from build123d import *

# Parameters (mm, degrees)
SKETCH1_R                    = 75.819
SKETCH1_R_2                  = 48.387
BOSS_EXTRUDE1_DEPTH          = 19.812
SKETCH2_R                    = 50.927
CUT_EXTRUDE1_DEPTH           = 8.7122
CHAMFER1_SIZE                = 0.762
SKETCH4_R                    = 4.2164
CUT_EXTRUDE2_DEPTH           = 20.812
CHAMFER2_SIZE                = 0.381
CIRPATTERN1_COUNT            = 16
CHAMFER2_OF_CIRPATTERN1_SIZE = 0.381
CUT_EXTRUDE3_DEPTH           = 0.79375


with BuildPart() as part:
    # Sketch1 → Boss-Extrude1 (new body)
    with BuildSketch(Plane(origin=(0, 0, 0), x_dir=(1, 0, 0), z_dir=(0, 1, 0))):
        Circle(SKETCH1_R)
        Circle(SKETCH1_R_2, mode=Mode.SUBTRACT)
    extrude(amount=BOSS_EXTRUDE1_DEPTH)

    # Sketch2 → Cut-Extrude1 (cut)
    with BuildSketch(Plane(origin=(0, 19.812, 0), x_dir=(1, 0, 0), z_dir=(0, 1, 0))):
        Circle(SKETCH2_R)
    extrude(amount=-CUT_EXTRUDE1_DEPTH, mode=Mode.SUBTRACT)

    # Chamfer1
    chamfer1_edges = [part.edges().sort_by_distance(p)[0] for p in [
        (-50.927, 19.812, 0),
        (-75.819, 0, 0),
        (-75.819, 19.812, 0),
    ]]
    chamfer(chamfer1_edges, length=CHAMFER1_SIZE)

    # Sketch3 → Cut-Revolve1 (revolve, cut)
    with BuildSketch(Plane.XY):
        Polygon((-60.325, 0), (-60.325, 1.6256), (-57.658, 0.6604), (-57.658, 1.27), (0, 1.27), (0, 0), align=None)
    revolve(axis=Axis((0, 19.812, 0), (0, -1, 0)), mode=Mode.SUBTRACT)

    # Sketch4 → Cut-Extrude2 (cut, through all)
    with BuildSketch(Plane(origin=(0, 19.812, 0), x_dir=(1, 0, 0), z_dir=(0, 1, 0))):
        with Locations((-12.705374275, 63.874229857)):
            Circle(SKETCH4_R)
    cut_extrude2 = extrude(amount=-CUT_EXTRUDE2_DEPTH, mode=Mode.SUBTRACT)

    # Chamfer2
    chamfer2_edges = [part.edges().sort_by_distance(p)[0] for p in [
        (-16.921774275, 0, -63.874229857),
        (-16.921774275, 19.812, -63.874229857),
    ]]
    chamfer(chamfer2_edges, length=CHAMFER2_SIZE)

    # CirPattern1: Cut-Extrude2 ×16 about axis
    cirpattern1_axis = Axis((0, 0, 0), (0, 1, 0))
    for i in range(1, CIRPATTERN1_COUNT):
        add(cut_extrude2.rotate(cirpattern1_axis, i * 360 / CIRPATTERN1_COUNT), mode=Mode.SUBTRACT)

    # Chamfer2 of CirPattern1
    chamfer2_of_cirpattern1_edges = [part.edges().sort_by_distance(p)[0] for p in [
        (-40.077290428, 0, -52.536410959),
        (-40.077290428, 19.812, -52.536410959),
        (-57.131402415, 0, -33.200399735),
        (-57.131402415, 19.812, -33.200399735),
        (-65.487776282, 0, -8.809928615),
        (-65.487776282, 19.812, -8.809928615),
        (-63.874229857, 0, 16.921774275),
        (-63.874229857, 19.812, 16.921774275),
        (-52.536410959, 0, 40.077290428),
        (-52.536410959, 19.812, 40.077290428),
        (-33.200399735, 0, 57.131402415),
        (-33.200399735, 19.812, 57.131402415),
        (-8.809928615, 0, 65.487776282),
        (-8.809928615, 19.812, 65.487776282),
        (16.921774275, 0, 63.874229857),
        (16.921774275, 19.812, 63.874229857),
        (40.077290428, 0, 52.536410959),
        (40.077290428, 19.812, 52.536410959),
        (57.131402415, 0, 33.200399735),
        (57.131402415, 19.812, 33.200399735),
        (65.487776282, 0, 8.809928615),
        (65.487776282, 19.812, 8.809928615),
        (63.874229857, 0, -16.921774275),
        (63.874229857, 19.812, -16.921774275),
        (52.536410959, 0, -40.077290428),
        (52.536410959, 19.812, -40.077290428),
        (33.200399735, 0, -57.131402415),
        (33.200399735, 19.812, -57.131402415),
        (8.809928615, 0, -65.487776282),
        (8.809928615, 19.812, -65.487776282),
    ]]
    chamfer(chamfer2_of_cirpattern1_edges, length=CHAMFER2_OF_CIRPATTERN1_SIZE)

    # Sketch5 → Cut-Extrude3 (cut, symmetric)
    with BuildSketch(Plane.XY):
        Polygon((-59.310240326, 0.913241856), (-75.819, 1.778429289), (-75.819, -2.195076128), (-59.310240326, -2.195076128), align=None)
        Polygon((59.310240326, 0.913241856), (59.310240326, -2.195076128), (75.819, -2.195076128), (75.819, 1.778429289), align=None)
    extrude(amount=CUT_EXTRUDE3_DEPTH, both=True, mode=Mode.SUBTRACT)


solid = part.part
Here's how the part is built. I have some questions about the finished solid (model axes, mm). A direction names the side the tool comes from. Round coordinates to 2 decimals unless told otherwise and drop trailing zeros. Order: outer loops, then holes, each group sorted by start corner. A loop starts at its lowest first (then second) coordinate and runs counter-clockwise, first axis right, second up. Notation, with made-up numbers: (-1, 85) -> (9, 85) arc R13 ccw to (9, 107) -> close; hole circle Ø7 at (-7.75, -3.5). An arc over 180 degrees is marked (long way). Return JSON: item names as keys, results as strings.
Q1. If we section it at A-A on x = 0: List the corners of the cut face in (y, z) for me (3 decimals), plus the area to 3 significant figures.
Filled sheet:
{"outline": "(0, -75.057) -> (0.762, -75.819) -> (19.05, -75.819) -> (19.812, -75.057) -> (19.812, -51.689) -> (19.05, -50.927) -> (11.1, -50.927) -> (11.1, -48.387) -> (1.27, -48.387) -> (1.27, -57.658) -> (0.66, -57.658) -> (1.626, -60.325) -> (0, -60.325) -> close; (0, 60.325) -> (1.626, 60.325) -> (0.66, 57.658) -> (1.27, 57.658) -> (1.27, 48.387) -> (11.1, 48.387) -> (11.1, 50.927) -> (19.05, 50.927) -> (19.812, 51.689) -> (19.812, 75.057) -> (19.05, 75.819) -> (0.762, 75.819) -> (0, 75.057) -> close", "area": "1,010 mm^2"}
Q2. If we section it at B-B on y = 13.75: Give the number of separate pieces and of enclosed holes in the cut face, plus the area to 3 significant figures.
Filled sheet:
{"separate pieces": "1", "enclosed holes": "17", "area": "9,020 mm^2"}
Q3. Which directions (+Z, -Z, +X, -X, +Y, -Y) give clear straight access to the entire face, cutting with the end or side of a thin tool? Please do faces 1 (the cylindrical face through (12.499, 0.969, 56.287)), 2 (the cylindrical face through (34.91, 10.04, -50.13)).
Filled sheet:
{"face 1": "-Y", "face 2": "+Y, -Y"}
Q4. I need wall thicknesses on line 1 along Z through (x, y) = (9, 3.5); line 2 along Z through (x, y) = (-62.5, 9.75); line 3 along X through (y, z) = (13.5, 14.5). Which ranges of each line are inside material? Lowest first, please. Write a range as from..to.
Filled sheet:
{"line 1": "z = -75.28..-65.89, -61.86..-47.54, 47.54..61.86, 65.89..75.28", "line 2": "z = -42.92..-16.69, -8.72..8.72, 16.69..42.92", "line 3": "x = -74.42..-67.69, -60.06..-48.82, 48.82..60.06, 67.69..74.42"}
Q5. If we mould it in two halves opening along X, with no side actions, what happens to faces 3 (the cylindrical face through (-54.148, 10.039, 31.965)), 4 (the conical face through (-1.64, 0.12, 75.16)), 5 (the cylindrical face through (59.76, 10.04, -13.62)), 6 (the flat face through (0, 0, -63))? For each: released by +X, released by -X, zero draft, split by the parting line, or undercut.
Filled sheet:
{"face 3": "undercut", "face 4": "split by the parting line", "face 5": "undercut", "face 6": "zero draft"}
Q6. For pin 1 Ø2 at (y, z) = (15, 3) entering from +X; pin 2 Ø13.5 at (x, z) = (-12.71, -63.87) entering from -Y; pin 3 Ø1.5 at (y, z) = (14, -27) entering from -X; pin 4 Ø6.5 at (x, z) = (36.18, 54.15) entering from +Y, each with a flat end and sliding along its axis, tell me the tip position at first contact or that it passes through.
Filled sheet:
{"pin 1": "stops at x = 75.79", "pin 2": "stops at y = 0", "pin 3": "stops at x = -71.13", "pin 4": "passes through"}
